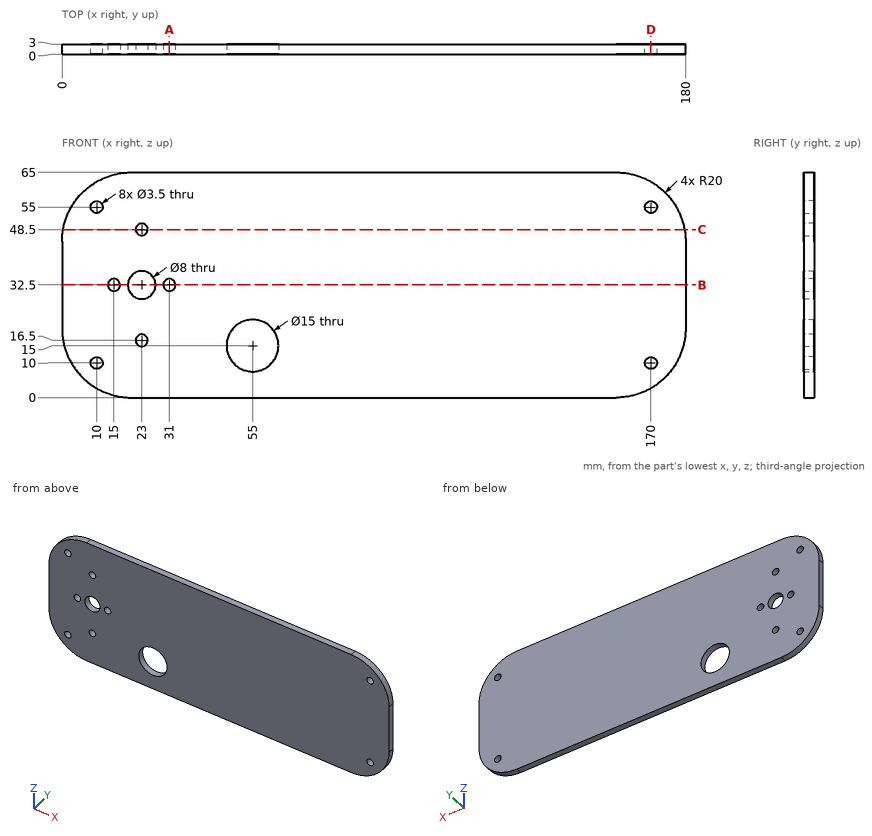
Here's the drawing with two shaded views (mm, measured from the low corner). I have some questions. Round coordinates to 2 decimals unless told otherwise and drop trailing zeros. Loops run counter-clockwise (first coordinate to the right, second up) from the corner with the lowest first, then second, coordinate; pieces in that order, holes last.
Item 1: Suppose I cut it at A-A, the plane x = 31. Write out the boundary of the cut face in (y, z), then the cut area to 4 significant figures.
Item 2: Suppose I cut it at D-D, the plane x = 170. Write out the boundary of the cut face in (y, z), then the cut area to 3 significant figures.
Item 3: Please list where these lines run through material, in increasing order: L1, parallel to X at y = 1.2, z = 32.5; L2, parallel to X at y = 1.25, z = 11; L3, parallel to Z at x = 10, y = 2.3.
Item 4: Suppose I cut it at C-C, the plane z = 48.5. Write out the boundary of the cut face in (x, y).
Item 5: Will this pin go through, and if not, where does the flat tip stop? pin 1 Ø5 at (x, z) = (122, 57.5) entering from -Y.
Item 6: Suppose I cut it at B-B, the plane z = 32.5. Write out the boundary of the cut face in (x, y).
Reported:
1. outline: (0, 0) - (3, 0) - (3, 30.75) - (0, 30.75) - close; (0, 34.25) - (3, 34.25) - (3, 65) - (0, 65) - close
1. area: 184.5 mm2
2. outline: (0, 2.68) - (3, 2.68) - (3, 8.25) - (0, 8.25) - close; (0, 11.75) - (3, 11.75) - (3, 53.25) - (0, 53.25) - close; (0, 56.75) - (3, 56.75) - (3, 62.32) - (0, 62.32) - close
2. area: 158 mm2
3. L1: x = 0 to 13.25, 16.75 to 19, 27 to 29.25, 32.75 to 180
3. L2: x = 2.14 to 8.56, 11.44 to 48.66, 61.34 to 168.56, 171.44 to 177.86
3. L3: z = 2.68 to 8.25, 11.75 to 53.25, 56.75 to 62.32
4. outline: (0.31, 0) - (21.25, 0) - (21.25, 3) - (0.31, 3) - close; (24.75, 0) - (179.69, 0) - (179.69, 3) - (24.75, 3) - close
5. pin 1: stops at y = 0
6. outline: (0, 0) - (13.25, 0) - (13.25, 3) - (0, 3) - close; (16.75, 0) - (19, 0) - (19, 3) - (16.75, 3) - close; (27, 0) - (29.25, 0) - (29.25, 3) - (27, 3) - close; (32.75, 0) - (180, 0) - (180, 3) - (32.75, 3) - close
